Autodesk Inventor part; units mm, degrees
ref_plane "YZ Plane" through (0, 0, 0) normal (1, 0, 0) x (0, 1, 0)
ref_plane "XZ Plane" through (0, 0, 0) normal (0, 1, 0) x (-1, 0, 0)
ref_plane "XY Plane" through (0, 0, 0) normal (0, 0, 1) x (1, 0, 0)
sketch "Szkic1" plane through (0, 0, 0) normal (0, 0, 1) x (1, 0, 0)
  line L0 (14.7767, -38.9659) -> (51.7767, -38.9659)
  line L1 (51.7767, -38.9659) -> (51.7767, -18.9659)
  line L2 (51.7767, -18.9659) -> (14.7767, -18.9659)
  line L3 (43.2767, -28.9659) -> (40.2767, -28.9659) construction
  line L4 (43.2767, -26.9659) -> (40.2767, -26.9659)
  line L5 (40.2767, -30.9659) -> (43.2767, -30.9659)
  arc A0 (43.2767, -30.9659) -> (43.2767, -26.9659) centre (43.2767, -28.9659) ccw
  arc A1 (40.2767, -26.9659) -> (40.2767, -30.9659) centre (40.2767, -28.9659) ccw
  line L6 (14.7767, -38.9659) -> (14.7767, -18.9659)
  line L7 (50.7767, -37.9659) -> (15.7767, -37.9659)
  line L8 (15.7767, -37.9659) -> (15.7767, -19.9659)
  line L9 (15.7767, -19.9659) -> (50.7767, -19.9659)
  line L10 (50.7767, -19.9659) -> (50.7767, -37.9659)
  line L11 (30.7767, -37.9659) -> (30.7767, -19.9659)
  point P0 (0, 0)
  point P1 (41.7767, -28.9659)
  dimension "d0" = 20
  dimension "d1" = 37
  dimension "d2" = 10
  dimension "d3" = 10
  dimension "d4" = 1.5
  dimension "d5" = 4
  dimension "d6" = 37
  dimension "d7" = 1
  dimension "d8" = 20
extrude "Wyciągnięcie proste1" add sketch "Szkic1" along normal blind 5 contours L7 L11 L9 L10 | L7 L8 L9 L11
extrude "Wyciągnięcie proste2" add sketch "Szkic1" against normal blind 15 contours L7 L8 L9 L11
chamfer "Faza1" distance 2 angle 45 2 edges at (50.7767, -19.9659, 2.5) (50.7767, -37.9659, 2.5)
fillet "Zaokrąglenie1" radius 3 2 edges at (15.7767, -37.9659, -5) (15.7767, -19.9659, -5)
sketch "Szkic2" plane through (0, 0, -15) normal (0, 0, -1) x (-1, 0, 0)
  arc A0 (-15.7767, -22.9659) -> (-18.7767, -19.9659) centre (-18.7767, -22.9659) ccw
  line L0 (-18.7767, -19.9659) -> (-30.7767, -19.9659)
  line L1 (-30.7767, -19.9659) -> (-30.7767, -37.9659)
  line L2 (-30.7767, -37.9659) -> (-18.7767, -37.9659)
  arc A1 (-18.7767, -37.9659) -> (-15.7767, -34.9659) centre (-18.7767, -34.9659) ccw
  line L3 (-15.7767, -34.9659) -> (-15.7767, -22.9659)
  point P0 (0, 0)
  point P1 (-23.2767, -28.9659)
  dimension "d17" = 18
  dimension "d18" = 15
  dimension "d19" = 7.5
  dimension "d20" = 9
hole "Otwór1" at (23.2767, -28.9659, -15) direction (0, 0, 1) diameter 4 end through all
fillet "Zaokrąglenie2" radius 1.5 2 edges at (30.7767, -37.9659, -7.5) (30.7767, -19.9659, -7.5)
equation "\"d6\" = d1"
properties part number "3DP_ABS_X_End_Bearing_Mount"
Build history of the part. All positions in model axes, mm. A direction names the side the tool comes from. Coordinates: 2 decimals unless noted, no trailing zeros. Order: outer loops, then holes, each group sorted by start corner. A loop starts at its lowest first (then second) coordinate and runs counter-clockwise, first axis right, second up. Notation, with made-up numbers: (75.25, -5.5) -> (117.25, -5.5) arc R6 ccw to (117.25, 2.5) -> close; hole circle Ø5 at (9.5, 4). An arc over 180 degrees is marked (long way). Answer in a Markdown table with one row per item. Add a question column.
Q1. Which spindle directions (+Z, -Z, +X, -X, +Y, -Y) get a long thin tool onto all of the face, cutting with end or side? Do faces 4 (the face through (30.326, -20.394, -7.605)), 5 (the face through (30.349, -37.515, -7.605)), 6 (the face through (38.277, -29.01, 2.465)), 7 (the face through (49.79, -20.98, 2.53)), 8 (the face through (30.777, -29, -7)). Say none if no direction does.
Q2. Band-saw the part on C-C, the plane z = -11.25. List the corners of the cut face in (x, y).
Q3. Mould opens along X. For faces 1 (the face through (15.777, -29, -5)), 2 (the face through (27, -19.966, -3)), 3 (the face through (42, -26.966, 2)) say: +X half, -X half, draft (parallel to the pull), parting line (faces both ways), or undercut.
Q4. Wall check: line 1 along X through (y, z) = (-30.5, 2.75); line 2 along X through (y, z) = (-27.5, 2.75); line 3 along Z through (x, y) = (33, -27.75). Give the ranges that are in metal, low to high. Write a range as [from, to].
Q5. Band-saw the part on A-A, the plane y = -24.5. List the corners of the cut face in (x, z), then the cut area to 3 significant figures.
Q6. Band-saw the part on B-B, the plane z = 1.25. List the corners of the cut face in (x, y), then the cut area to 3 significant figures.
Q7. Band-saw the part on D-D, the plane x = 33. List the corners of the cut face in (y, z).
Q8. Drop a flat-ended pin along its axis: pin 1 (2 mm diameter, centred on x = 43, y = -26, fed in from -Z). Give the stop position or say it passes through.
Answers follow:
| question | item | result |
|---|---|---|
| 1 | face 4 | -Z, +X, +Y |
| 1 | face 5 | -Z, +X, -Y |
| 1 | face 6 | +Z, -Z |
| 1 | face 7 | +Z, -Z, +X, +Y |
| 1 | face 8 | -Z, +X, +Y, -Y |
| 2 | outline | (15.78, -34.97) arc R3 ccw to (18.78, -37.97) -> (29.28, -37.97) arc R1.5 ccw to (30.78, -36.47) -> (30.78, -21.47) arc R1.5 ccw to (29.28, -19.97) -> (18.78, -19.97) arc R3 ccw to (15.78, -22.97) -> close; hole circle Ø4 at (23.28, -28.97) |
| 3 | face 1 | -X half |
| 3 | face 2 | draft |
| 3 | face 3 | undercut |
| 4 | line 1 | [15.78, 21.99], [24.56, 38.99], [44.56, 50.78] |
| 4 | line 2 | [15.78, 21.92], [24.64, 38.92], [44.64, 50.78] |
| 4 | line 3 | [0, 5] |
| 5 | outline | (15.78, -15) -> (30.78, -15) -> (30.78, 0) -> (50.78, 0) -> (50.78, 5) -> (15.78, 5) -> close |
| 5 | area | 400 mm^2 |
| 6 | outline | (15.78, -34.97) arc R3 ccw to (18.78, -37.97) -> (48.78, -37.97) -> (50.78, -35.97) -> (50.78, -21.97) -> (48.78, -19.97) -> (18.78, -19.97) arc R3 ccw to (15.78, -22.97) -> close; hole circle Ø4 at (23.28, -28.97); hole (40.28, -30.97) -> (43.28, -30.97) arc R2 ccw to (43.28, -26.97) -> (40.28, -26.97) arc R2 ccw to start |
| 6 | area | 585 mm^2 |
| 7 | outline | (-37.97, 0) -> (-19.97, 0) -> (-19.97, 5) -> (-37.97, 5) -> close |
| 8 | pin 1 | z = 0 |
